```python
from build123d import *

# Parameters (mm, degrees)
F0_R            = 44.45
F0_R_2          = 38.1
F1_DEPTH        = 127
F2_W            = 6.35
F2_H            = 5.1593752402
F3_DEPTH        = 10.16
F3_COPIES_COUNT = 3


# Not quite as in the source:
# - a pattern or mirror of a feature is missing from the dataset's text; its kind, count and spacing are read off the source's solid


with BuildPart() as f1:
    # F0 (on Top) → F1 (new body)
    with BuildSketch(Plane.XY):
        Circle(F0_R)
        Circle(F0_R_2, mode=Mode.SUBTRACT)
    extrude(amount=F1_DEPTH)

    # F2 (on Top) → F3 (join)
    with BuildSketch(Plane.XY):
        with Locations((-34.925, 0)):
            Rectangle(F2_W, F2_H)
    f3 = extrude(amount=F3_DEPTH)

    # F3_copies: F3 ×3 about axis
    f3_copies_axis = Axis((0, 0, 0), (0, 0, 1))
    for i in range(1, F3_COPIES_COUNT):
        add(f3.rotate(f3_copies_axis, i * 360 / F3_COPIES_COUNT))


solid = f1.part
```
Model file for the job. Use its own axes, mm. A direction names the side the tool comes from. Coordinates: 2 decimals unless noted, no trailing zeros. Write each loop counter-clockwise with the first axis right and the second up, starting at its lowest first coordinate (ties: lowest second). Pieces come first, ordered by that corner, then holes. Notation, with made-up numbers: (89, -28) - (117, -28) arc R19 ccw to (117, -15) - close; hole circle Ø3 at (47.5, 18.5). An arc over 180 degrees is marked (long way). One line per question, with ' | ' between items. Start each with the question number.
Q1. Drill centre lines: line 1 (Y direction, x = 0, z = 95); line 2 (Y direction, x = 21, z = 48); line 3 (X direction, y = -16, z = 92). Where is each one in solid material? Low to high. Write a range as [from, to].
Q2. Cut at A-A, the plane x = 0. List the corners of the cut face in (y, z).
Q3. Pin check, flat tips, straight feed: pin 1 (3 mm diameter, centred on y = 13, z = 69, fed in from +X); pin 2 (1 mm diameter, centred on x = -31.5, z = 32.5, fed in from +Y); pin 3 (2.5 mm diameter, centred on x = 18.5, y = -28.5, fed in from +Z). Stop position of each tip, or through.
Q4. Cut at B-B, the plane y = 0. List the corners of the cut face in (x, z).
Q5. Cut at C-C, the plane z = 93. List the corners of the cut face in (x, y), then the cut area to 3 significant figures.
Q6. 3-axis set-ups, long thin cutter, end or side, ignore diameter. For faces 4 (the face through (33, 20, 127)), 5 (the face through (-31.75, 0, 5)), 6 (the face through (18, 30, 10.16)): which of +Z, -Z, +X, -X, +Y, -Y reach the whole face in a straight line?
Q7. Pull direction Y, two halves, no side cores. Call faces 1 (the face through (42.397, 13.352, 62.611)), 2 (the face through (-33, 0, 0)), 3 (the face through (15.23, 31.54, 5.01)): pulls with the +Y half, pulls with the -Y half, needs draft (parallel to the pull), parting line crosses it, or undercut.
Q8. Cut at D-D, the plane x = -25. List the corners of the cut face in (y, z), then the cut area to 3 significant figures.
Answer below:
1) line 1: [-44.45, -38.1], [38.1, 44.45] | line 2: [-39.18, -31.79], [31.79, 39.18] | line 3: [-41.47, -34.58], [34.58, 41.47]
2) outline: (-44.45, 0) - (-38.1, 0) - (-38.1, 127) - (-44.45, 127) - close; (38.1, 0) - (44.45, 0) - (44.45, 127) - (38.1, 127) - close
3) pin 1: x = 42.94 | pin 2: y = 31.86 | pin 3: z = 10.16
4) outline: (-44.45, 0) - (-31.75, 0) - (-31.75, 10.16) - (-38.1, 10.16) - (-38.1, 127) - (-44.45, 127) - close; (38.1, 0) - (44.45, 0) - (44.45, 127) - (38.1, 127) - close
5) outline: circle Ø88.9 at (0, 0); hole circle Ø76.2 at (0, 0) | area: 1,650 mm^2
6) face 4: +Z, +X, -X, +Y, -Y | face 5: +Z, -Z | face 6: +Z
7) face 1: parting line crosses it | face 2: needs draft | face 3: undercut
8) outline: (-36.75, 0) - (-28.75, 0) - (-28.75, 127) - (-36.75, 127) - close; (28.75, 0) - (36.75, 0) - (36.75, 127) - (28.75, 127) - close | area: 2,030 mm^2
